from build123d import *

# Parameters (mm, degrees)
AUFSATZ_LINEAR_AUSTRAGEN1_DEPTH      = 6
SCHNITT_LINEAR_AUSTRAGEN1_DEPTH      = 72.169611735
SCHNITT_LINEAR_AUSTRAGEN1_DEPTH_BACK = 72.169611735
SCHNITT_LINEAR_AUSTRAGEN2_DEPTH      = 72.169611735
SCHNITT_LINEAR_AUSTRAGEN2_DEPTH_BACK = 72.169611735
AUFSATZ_LINEAR_AUSTRAGEN2_DEPTH      = 4
SCHNITT_LINEAR_AUSTRAGEN3_DEPTH      = 72.169611735
SCHNITT_LINEAR_AUSTRAGEN3_DEPTH_BACK = 72.169611735
SKIZZE7_R                            = 1.05
SCHNITT_LINEAR_AUSTRAGEN4_DEPTH      = 5


with BuildPart() as part:
    # Skizze1 → Aufsatz-Linear austragen1 (new body)
    with BuildSketch(Plane(origin=(0, 0, 0), x_dir=(1, 0, 0), z_dir=(0, 1, 0))):
        with BuildLine():
            Line((9.557167706, 20.388739502), (6.321745697, -70))
            Line((6.321745697, -70), (5.021745697, -70))
            Line((5.021745697, -70), (4.552285436, -65.533383981))
            Line((4.552285436, -65.533383981), (1.752285436, -65.533383981))
            Line((1.752285436, -65.533383981), (1.282825175, -70))
            Line((1.282825175, -70), (-2.768942942, -70))
            Line((-2.768942942, -70), (-3.238403203, -65.533383981))
            Line((-3.238403203, -65.533383981), (-6.038403203, -65.533383981))
            Line((-6.038403203, -65.533383981), (-6.507863464, -70))
            Line((-6.507863464, -70), (-8.17258631, -70))
            Line((-8.17258631, -70), (-11.362818073, 19.126249046))
            ThreePointArc((-11.362818073, 19.126249046), (-8.433885885, 26.197316858), (-1.362818073, 29.126249046))
            Line((-1.362818073, 29.126249046), (-0.362818073, 29.126249046))
            ThreePointArc((-0.362818073, 29.126249046), (6.24683757, 26.630411376), (9.557167706, 20.388739502))
        make_face()
    extrude(amount=AUFSATZ_LINEAR_AUSTRAGEN1_DEPTH)

    # Skizze3 → Schnitt-Linear austragen1 (cut, two sides: drawn at the far end of the back side and taken through both)
    with BuildSketch(Plane(origin=(0, 0, 0), x_dir=(0, 0, -1), z_dir=(1, 0, 0)).offset(-SCHNITT_LINEAR_AUSTRAGEN1_DEPTH_BACK)):
        Polygon((16.673690486, 6), (-70, 6), (-70, 2.973288034), align=None)
    extrude(amount=SCHNITT_LINEAR_AUSTRAGEN1_DEPTH + SCHNITT_LINEAR_AUSTRAGEN1_DEPTH_BACK, mode=Mode.SUBTRACT)

    # Skizze4 → Schnitt-Linear austragen2 (cut, two sides: drawn at the far end of the back side and taken through both)
    with BuildSketch(Plane(origin=(0, 0, 0), x_dir=(0, 0, -1), z_dir=(1, 0, 0)).offset(-SCHNITT_LINEAR_AUSTRAGEN2_DEPTH_BACK)):
        Polygon((20.388739502, 6), (29.126249046, 4.459341323), (29.126249046, 6), align=None)
    extrude(amount=SCHNITT_LINEAR_AUSTRAGEN2_DEPTH + SCHNITT_LINEAR_AUSTRAGEN2_DEPTH_BACK, mode=Mode.SUBTRACT)

    # Skizze5 → Aufsatz-Linear austragen2 (add)
    with BuildSketch(Plane.XZ):
        with BuildLine():
            Line((-7.933885885, -12.055181234), (-7.933885885, -3.371441204))
            Line((-7.933885885, -3.371441204), (6.208249739, -3.371441204))
            Line((6.208249739, -3.371441204), (6.208249739, -12.055181234))
            ThreePointArc((6.208249739, -12.055181234), (-0.862818073, -29.126249046), (-7.933885885, -12.055181234))
        make_face()
    extrude(amount=AUFSATZ_LINEAR_AUSTRAGEN2_DEPTH)

    # Skizze6 → Schnitt-Linear austragen3 (cut, two sides: drawn at the far end of the back side and taken through both)
    with BuildSketch(Plane(origin=(0, 0, 0), x_dir=(0, 0, -1), z_dir=(1, 0, 0)).offset(-SCHNITT_LINEAR_AUSTRAGEN3_DEPTH_BACK)):
        Polygon((12.066816312, -1.992514478), (29.126249046, 1.945965899), (29.126249046, -4), (3.371441204, -4), (3.371441204, -2), align=None)
    extrude(amount=SCHNITT_LINEAR_AUSTRAGEN3_DEPTH + SCHNITT_LINEAR_AUSTRAGEN3_DEPTH_BACK, mode=Mode.SUBTRACT)

    # Skizze7 → Schnitt-Linear austragen4 (cut)
    with BuildSketch(Plane(origin=(0, -4.536559366, -1.047347255), x_dir=(1, 0, 0), z_dir=(0, -0.9743700647852368, -0.22495105434385881))):
        with Locations(Location((-0.862818073, -14.009326359, 0), (0, 0, 270))):
            Circle(SKIZZE7_R)
        with Locations(Location((-0.862818073, -17.909326359, 0), (0, 0, 270))):
            Circle(SKIZZE7_R)
        with Locations(Location((-0.862818073, -21.809326359, 0), (0, 0, 270))):
            Circle(SKIZZE7_R)
        with Locations(Location((-0.862818073, -25.709326359, 0), (0, 0, 270))):
            Circle(SKIZZE7_R)
    extrude(amount=-SCHNITT_LINEAR_AUSTRAGEN4_DEPTH, mode=Mode.SUBTRACT)


solid = part.part
Part model, mm, in its own coordinate system. A direction names the side the tool comes from. Round coordinates to 2 decimals unless told otherwise and drop trailing zeros. Write each loop counter-clockwise with the first axis right and the second up, starting at its lowest first coordinate (ties: lowest second). Pieces come first, ordered by that corner, then holes. Notation, with made-up numbers: M 58,-2.5 L 96,-2.5 A20 ccw 96,22.5 Z; hole C 36,66 d8. An arc over 180 degrees is marked long. Return JSON: item names as keys, results as strings. Group by question number.
(1) Saw through at A-A on x = 3. Write the cut outline in (y, z).
(2) Drill centre lines: probe 1 along Z at (x, y) = (-1.5, 0.5); probe 2 along X at (y, z) = (1, -21.5); probe 3 along X at (y, z) = (2, -11.5). Where is each one in solid material? Low to high.
(3) Saw through at B-B on z = -9.5. Write the cut outline in (x, y).
(4) Two-plate mould, pull along Z, no slides. Class faces 1 (the face through (3, 2, 65.533)), 2 (the face through (-1.01, -0.05, -20.48)), 3 (the face through (-0.848, 3.483, -13.559)): +Z half, -Z half, draft (parallel to the pull), parting line (faces both ways), or undercut.
(5) Pin check, flat tips, straight feed: pin 1 Ø4 at (x, z) = (0.5, 8.5) entering from -Y; pin 2 Ø1.4 at (x, y) = (-4, 1.5) entering from +Z; pin 3 Ø4 at (y, z) = (2, 50.5) entering from +X; pin 4 Ø1 at (x, z) = (7.5, 56) entering from -Y. Stop position of each tip, or through.
(6) Which spindle directions (+Z, -Z, +X, -X, +Y, -Y) get a long thin tool onto all of the face, cutting with end or side? Do faces 4 (the face through (-0.85, 4.36, -17.36)), 5 (the face through (-1, -1, -3.371)), 6 (the face through (-1, 6, -19)), 7 (the face through (-6.27, 1.54, 67.74)), 8 (the face through (6.208, -1, -8)). Say none if no direction does.
(7) Saw through at D-D on z = 32. Write the cut outline in (x, y), then the cut area to 3 significant figures.
Returned:
{
 "1": {"outline": "M -2,-3.37 L -1.99,-12.07 L 1.81,-28.54 L 4.56,-28.54 L 6,-20.39 L 6,-16.67 L 3.13,65.53 L 0,65.53 L 0,-3.37 Z"},
 "2": {"probe 1": "-21.41 to -19.12, -17.41 to -15.12, -13.41 to 70", "probe 2": "-11.08 to -1.7, -0.03 to 9.35", "probe 3": "-11.09 to 9.24"},
 "3": {"outline": "M -11.02,0 L -7.93,0 L -7.93,-1.99 L 6.21,-1.99 L 6.21,0 L 9.17,0 L 9.17,5.75 L -11.02,5.75 Z"},
 "4": {"face 1": "+Z half", "face 2": "-Z half", "face 3": "undercut"},
 "5": {"pin 1": "y = 0", "pin 2": "z = 65.53", "pin 3": "x = 7.09", "pin 4": "through"},
 "6": {"face 4": "none", "face 5": "+Z, +X, -X, -Y", "face 6": "+Z, -Z, +X, -X, +Y", "face 7": "+Z, +Y, -Y", "face 8": "+Z, +X, -Y"},
 "7": {"outline": "M -9.53,0 L 7.68,0 L 7.68,4.3 L -9.53,4.3 Z", "area": "74.0 mm²"}
}
